from build123d import *

# Parameters (mm, degrees)
F1_DEPTH = 16
F3_D     = 5
F4_W     = 1
F4_H     = 16
F5_DEPTH = 1
F6_W     = 1
F6_H     = 16
F7_DEPTH = 1


# Not quite as in the source:
# - a feature names something its author has since deleted; it is built from what else it names


with BuildPart() as f1:
    # F0 (on Front) → F1 (new body)
    with BuildSketch(Plane.XZ):
        with BuildLine():
            Line((-21, 8), (-21, -8))
            Line((-21, -8), (-16, -8))
            ThreePointArc((-16, -8), (-9, -1), (-2, -8))
            Line((-2, -8), (12.0004845034, -8))
            ThreePointArc((12.0004845034, -8), (10.125, 0), (12.0004845034, 8))
            Line((12.0004845034, 8), (-2, 8))
            ThreePointArc((-2, 8), (-9, 1), (-16, 8))
            Line((-16, 8), (-21, 8))
        make_face()
    extrude(amount=F1_DEPTH)

    # F3 (through all)
    with Locations(Plane.XY.offset(8)):
        with Locations((5, -8)):
            Hole(F3_D / 2)

    # F4 (on face) → F5 (cut)
    with BuildSketch(Plane.XY.offset(8)):
        with Locations((-18.5, -8)):
            Rectangle(F4_W, F4_H)
    extrude(amount=-F5_DEPTH, mode=Mode.SUBTRACT)

    # F6 (on face) → F7 (join)
    with BuildSketch(Plane(origin=(0, 0, -8), x_dir=(1, 0, 0), z_dir=(0, 0, -1))):
        with Locations((-18.5, 8)):
            Rectangle(F6_W, F6_H)
    extrude(amount=F7_DEPTH)


solid = f1.part
Geometry: final body of the model. Coordinates: model frame, mm. A direction names the side the tool comes from. Give positions to 0.01 mm unless a question says otherwise; leave off trailing zeros. Write each loop counter-clockwise with the first axis right and the second up, starting at its lowest first coordinate (ties: lowest second). Pieces come first, ordered by that corner, then holes.
(1) First-contact query: P1, Ø1.5, axis at x = -6.5, y = -12.5, coming from the -Z side; P2, Ø1, axis at y = -2, z = 6, coming from the +X side; P3, Ø3, axis at x = -9.5, y = -6, coming from the -Z side; P4, Ø4, axis at x = 5, y = -8, coming from the +Z side. Flat tips, straight axial feed; report the tip coordinate or a pass-through.
(2) Cut plane D-D, the plane y = -13.5. Return loops of the section in (x, z) (3 decimals).
(3) Access query for faces 5 (the flat face through (3, -6, -8)), 6 (the flat face through (-19, -8.1, 7.5)), 7 (the flat face through (-18.5, -8.1, -9)). Directions: +Z, -Z, +X, -X, +Y, -Y. A direction counts if a zero-diameter tool reaches every point of the face in a straight line with its end or side. Return the directions, or none.
(4) Ray query, line 1 (Y direction, x = 5, z = 3.75); line 2 (X direction, y = -6.25, z = 6.25); line 3 (Z direction, x = -17, y = -11.5). Return the intervals inside material, ascending.
(5) Cut plane B-B, the plane y = -6. Return loops of the section in (x, z) (3 decimals), then the cut area to 3 significant figures.
(6) Cut plane C-C, the plane z = -4. Return loops of the section in (x, y).
(7) Cut plane A-A, the plane x = 5. Return loops of the section in (y, z).
(8) Mould query, pull axis X, two halves, no side actions, for faces 1 (the flat face through (-20, -8, -8)), 2 (the cylindrical face through (3.85, -10.22, -0.11)), 3 (the cylindrical face through (-9, -8, 1)), 4 (the flat face through (-19, -7.9, -8.5)). Classes: released by +X, released by -X, zero draft, split by the parting line, or undercut.
Values follow:
1. P1: stops at z = -1.8
1. P2: stops at x = 11.34
1. P3: stops at z = -1.29
1. P4: passes through
2. outline: (-21, -8) - (-19, -8) - (-19, -9) - (-18, -9) - (-18, -8) - (-16, -8) arc R7 cw to (-2, -8) - (12, -8) arc R18 cw to (12, 8) - (-2, 8) arc R7 cw to (-16, 8) - (-18, 8) - (-18, 7) - (-19, 7) - (-19, 8) - (-21, 8) - close
3. face 5: -Z, +X, +Y, -Y
3. face 6: +Z, +Y, -Y
3. face 7: -Z, +X, -X, +Y, -Y
4. line 1: y = -16 to -10.5, -5.5 to 0
4. line 2: x = -21 to -15.78, -2.22 to 3.21, 6.79 to 11.24
4. line 3: z = -8 to 8
5. outline: (-21, -8) - (-19, -8) - (-19, -9) - (-18, -9) - (-18, -8) - (-16, -8) arc R7 cw to (-2, -8) - (3.5, -8) - (3.5, 8) - (-2, 8) arc R7 cw to (-16, 8) - (-18, 8) - (-18, 7) - (-19, 7) - (-19, 8) - (-21, 8) - close; (6.5, -8) - (12, -8) arc R18 cw to (12, 8) - (6.5, 8) - close
5. area: 306 mm2
6. outline: (-21, -16) - (-14.74, -16) - (-14.74, 0) - (-21, 0) - close; (-3.26, -16) - (10.58, -16) - (10.58, 0) - (-3.26, 0) - close; hole circle Ø5 at (5, -8)
7. outline: (-16, -8) - (-10.5, -8) - (-10.5, 8) - (-16, 8) - close; (-5.5, -8) - (0, -8) - (0, 8) - (-5.5, 8) - close
8. face 1: zero draft
8. face 2: undercut
8. face 3: undercut
8. face 4: released by -X
